Could you check a few things on this model? Use its own coordinates, in mm. Give positions to 0.01 mm unless a question says otherwise; leave off trailing zeros. Write each loop counter-clockwise with the first axis right and the second up, starting at its lowest first coordinate (ties: lowest second). Pieces come first, ordered by that corner, then holes. Notation, with made-up numbers: M -31,6.25 L 16,6.25 A17 ccw 16,34.25 Z; hole C 25.5,0.5 d7. An arc over 180 degrees is marked long. Use one line per item in the form item = value.
from build123d import *

# Parameters (mm, degrees)
F1_DEPTH = 27.686


with BuildPart() as f1:
    # F0 (on Front) → F1 (new body)
    with BuildSketch(Plane.XZ):
        with BuildLine():
            Line((-34.980499, 7.33363), (-34.980499, 0))
            Line((-34.980499, 0), (0, 0))
            Line((0, 0), (-8.416646, 29.294888))
            ThreePointArc((-8.416646, 29.294888), (-17.393594, 42.452943), (-32.440795, 47.678049))
            Line((-32.440795, 47.678049), (-34.980499, 47.716875))
            Line((-34.980499, 47.716875), (-34.980499, 37.81363))
            ThreePointArc((-34.980499, 37.81363), (-24.204191, 33.349937), (-19.740499, 22.57363))
            ThreePointArc((-19.740499, 22.57363), (-24.204191, 11.797322), (-34.980499, 7.33363))
        make_face()
    extrude(amount=F1_DEPTH)


solid = f1.part
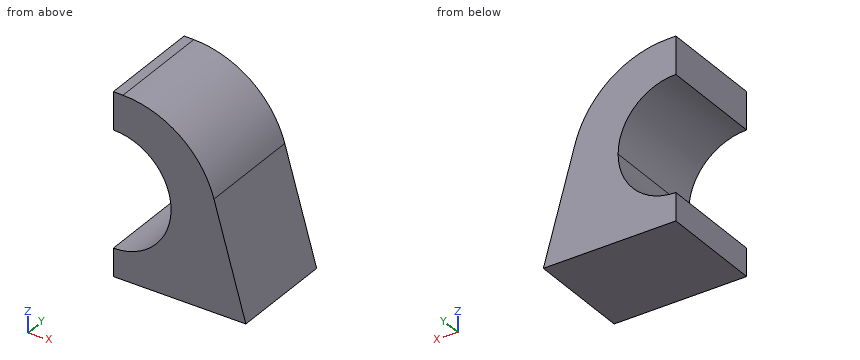
1) For pin 1 Ø6 at (x, y) = (-21.5, -13) entering from +Z; pin 2 Ø3 at (y, z) = (-18.5, 36) entering from +X; pin 3 Ø1 at (y, z) = (-6.5, 28.5) entering from +X; pin 4 Ø2 at (x, z) = (-5, 26) entering from -Y, each with a flat end and sliding along its axis, tell me the tip position at first contact or that it passes through.
Checked values:
pin_1 = 46.28
pin_2 = -10.56
pin_3 = -8.04
pin_4 = through
2) If I drill on L1, parallel to Z at x = -22, y = -7.75; L2, parallel to Z at x = -23, y = -4.5; L3, parallel to X at y = -24.25, z = 30, over which ranges is the centre line in solid material (lowest first)?
Checked values:
L1 = 0 to 14.59, 30.56 to 45.26
L2 = 0 to 13.15, 31.99 to 45.7
L3 = -21.67 to -8.63
3) I want a section at B-B, the plane y = -6. Please give me the cut outline in (x, z), plus the area to 3 significant figures.
Checked values:
outline = M -34.98,0 L 0,0 L -8.42,29.29 A25.4 ccw -32.44,47.68 L -34.98,47.72 L -34.98,37.81 A15.24 cw -19.74,22.57 A15.24 cw -34.98,7.33 Z
area = 907 mm2
4) I want a section at C-C, the plane x = -24.5. Please give me the cut outline in (y, z), plus the area to 3 significant figures.
Checked values:
outline = M -27.69,0 L 0,0 L 0,11.51 L -27.69,11.51 Z; M -27.69,33.64 L 0,33.64 L 0,46.28 L -27.69,46.28 Z
area = 669 mm2
5) I want a section at D-D, the plane z = 14.5. Please give me the cut outline in (x, y), plus the area to 3 significant figures.
Checked values:
outline = M -22.05,-27.69 L -4.17,-27.69 L -4.17,0 L -22.05,0 Z
area = 495 mm2
6) I want a section at A-A, the plane x = -30.5. Please give me the cut outline in (y, z), plus the area to 3 significant figures.
Checked values:
outline = M -27.69,0 L 0,0 L 0,8.01 L -27.69,8.01 Z; M -27.69,37.14 L 0,37.14 L 0,47.57 L -27.69,47.57 Z
area = 511 mm2
